from build123d import *

# Parameters (mm, degrees)
F0_R     = 15
F0_R_2   = 10
F1_DEPTH = 10


# Not quite as in the source:
# - ends of sketch curves that miss each other by under 0.0002 mm in the source are joined


with BuildPart() as f1:
    # F0 (on Front) → F1 (new body)
    with BuildSketch(Plane.XZ):
        with BuildLine():
            ThreePointArc((-77.8194442075, 29.4897614533), (-44.7134784315, 17.2871063454), (-18.8426622217, -6.704780414))
            ThreePointArc((-18.8426622217, -6.704780414), (-1.8148984382, -19.9174833666), (17.3205080757, -10))
            Line((17.3205080757, -10), (17.2196907343, -9.9417930808))
            Line((17.2196907343, -9.9417930808), (18.301055835, -8.0666818038))
            Line((18.301055835, -8.0666818038), (65.8985825054, 74.4684942965))
            ThreePointArc((65.8985825054, 74.4684942965), (66.2472754238, 74.9395201306), (66.5820179406, 75.4205601863))
            ThreePointArc((66.5820179406, 75.4205601863), (69.4871465026, 91.102664953), (60, 103.9230484541))
            ThreePointArc((60, 103.9230484541), (-25.9727536726, 117.1555208544), (-98.2982453147, 68.8291723621))
            ThreePointArc((-98.2982453147, 68.8291723621), (-99.9947150369, 42.9460461225), (-77.8194442075, 29.4897614533))
        make_face()
        with BuildLine():
            ThreePointArc((8.590003141, 5.1197505835), (9.6410588477, 2.655180652), (10, 0))
            ThreePointArc((10, 0), (-9.6410588477, -2.655180652), (8.590003141, 5.1197505835))
        make_face(mode=Mode.SUBTRACT)
        with Locations((-77.8194442075, 54.4897614533)):
            Circle(F0_R, mode=Mode.SUBTRACT)
        with BuildLine():
            Line((44.4926580322, 67.3757573805), (13.9195380637, 14.3612833721))
            ThreePointArc((13.9195380637, 14.3612833721), (-1.1386278406, 19.9675618602), (-15.461870052, 12.6858414973))
            ThreePointArc((-15.461870052, 12.6858414973), (-34.2806761155, 28.431524103), (-56.2400022895, 39.3796735521))
            ThreePointArc((-56.2400022895, 39.3796735521), (-56.8984637414, 39.6141223401), (-57.5584712538, 39.84418277))
            ThreePointArc((-57.5584712538, 39.84418277), (-57.4489819567, 39.9968574072), (-57.3406431002, 40.1503505446))
            ThreePointArc((-57.3406431002, 40.1503505446), (-54.0993659231, 62.3864624217), (-70.0220352349, 78.2426647141))
            ThreePointArc((-70.0220352349, 78.2426647141), (-20.6376982657, 102.9518596738), (34.4547303835, 99.1860451586))
            ThreePointArc((34.4547303835, 99.1860451586), (30.9270685064, 80.5839621211), (44.4926580322, 67.3757573805))
        make_face(mode=Mode.SUBTRACT)
        with Locations((50, 86.6025403784)):
            Circle(F0_R_2, mode=Mode.SUBTRACT)
        with BuildLine():
            Line((17.2196907343, -9.9417930808), (17.3205080757, -10))
            ThreePointArc((17.3205080757, -10), (17.836994805, -9.0466356358), (18.301055835, -8.0666818038))
            Line((18.301055835, -8.0666818038), (17.2196907343, -9.9417930808))
        make_face()
        with BuildLine():
            ThreePointArc((18.301055835, -8.0666818038), (17.836994805, -9.0466356358), (17.3205080757, -10))
            Line((17.3205080757, -10), (66.5820179406, 75.4205601863))
            ThreePointArc((66.5820179406, 75.4205601863), (66.2472754238, 74.9395201306), (65.8985825054, 74.4684942965))
            Line((65.8985825054, 74.4684942965), (18.301055835, -8.0666818038))
        make_face()
    extrude(amount=F1_DEPTH)


solid = f1.part
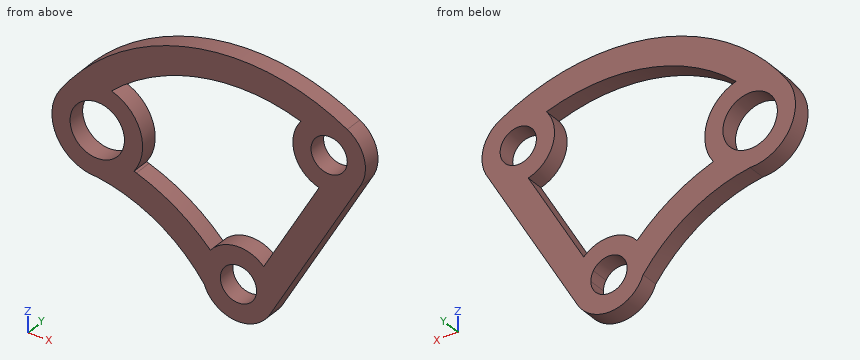
Work out the finished part from the listing and answer in its coordinate system (mm). Round coordinates to 2 decimals unless told otherwise and drop trailing zeros. Write each loop counter-clockwise with the first axis right and the second up, starting at its lowest first coordinate (ties: lowest second). Pieces come first, ordered by that corner, then holes. Notation, with made-up numbers: (58, 7.5) - (82, 7.5) arc R26 cw to (82, 22.5) - close; hole circle Ø1 at (71, 5). An arc over 180 degrees is marked (long way). Answer in a Markdown table with one row per item. Add a question column.
1. A cutting plane is placed at A-A, the plane x = -2. Determine the outline of the cut face in (y, z), and give its area (3 significant figures).
2. A cutting plane is placed at B-B, the plane z = 37.5. Determine the outline of the cut face in (x, y).
3. A cutting plane is placed at C-C, the plane x = 50. Determine the outline of the cut face in (y, z).
4. A cutting plane is placed at D-D, the plane y = -1.75. Determine the outline of the cut face in (x, z).
5. Given pin 1 (4 mm diameter, centred on x = 26, y = -7, fed in from -Z); pin 2 (3 mm diameter, centred on y = -8, z = 0, fed in from -X); pin 3 (2 mm diameter, centred on y = -8, z = 12, fed in from -X), each flat-ended and moving along its own axis, determine where each tip first touches the part or whether it passes through.
6. Find the intervals of material crossed by line 1 along X through (y, z) = (-7.25, 50); line 2 along X through (y, z) = (-3.25, 78.5); line 3 along Z through (x, y) = (1, -2.25), in increasing order. Write a range as from..to.
Worked out:
| question | item | result |
|---|---|---|
| 1 | outline | (-10, -19.9) - (0, -19.9) - (0, -9.8) - (-10, -9.8) - close; (-10, 9.8) - (0, 9.8) - (0, 19.9) - (-10, 19.9) - close; (-10, 104.98) - (0, 104.98) - (0, 119.98) - (-10, 119.98) - close |
| 1 | area | 352 mm^2 |
| 2 | outline | (-96.16, -10) - (-51.4, -10) - (-51.4, 0) - (-96.16, 0) - close; (27.26, -10) - (44.71, -10) - (44.71, 0) - (27.26, 0) - close |
| 3 | outline | (-10, 46.67) - (0, 46.67) - (0, 76.6) - (-10, 76.6) - close; (-10, 96.6) - (0, 96.6) - (0, 109.09) - (-10, 109.09) - close |
| 4 | outline | (-98.3, 68.83) arc R25 ccw to (-77.82, 29.49) arc R90 cw to (-18.84, -6.7) arc R20 ccw to (17.33, -9.98) - (66.58, 75.42) arc R20 ccw to (60, 103.92) arc R120 ccw to start; hole circle Ø30 at (-77.82, 54.49); hole (-70.02, 78.24) arc R25 cw to (-57.56, 39.84) arc R105 cw to (-56.24, 39.38) arc R105 cw to (-15.46, 12.69) arc R20 cw to (13.92, 14.36) - (44.49, 67.38) arc R20 cw to (34.45, 99.19) arc R105 ccw to start; hole circle Ø20 at (0, 0); hole circle Ø20 at (50, 86.6) |
| 5 | pin 1 | z = 1.58 |
| 5 | pin 2 | x = -25.54 |
| 5 | pin 3 | x = -38.35 |
| 6 | line 1 | -102.41..-92.13, -63.51..-53.23, 34.47..51.92 |
| 6 | line 2 | -90.76..-69.73, 31.71..44.14, 55.86..68.29 |
| 6 | line 3 | -19.97..-9.95, 9.95..19.97, 105..120 |
